```python
from build123d import *

# Parameters (mm, degrees)
BOSS_EXTRUDE1_DEPTH     = 60
CUT_EXTRUDE1_DEPTH      = 144.527000944
CUT_EXTRUDE1_DEPTH_BACK = 3
SKETCH3_R               = 2
CUT_EXTRUDE2_DEPTH      = 4


with BuildPart() as part:
    # Sketch1 → Boss-Extrude1 (new body)
    with BuildSketch(Plane(origin=(0, 0, 0), x_dir=(1, 0, 0), z_dir=(0, 1, 0))):
        Polygon((130, 10), (0, 10), (10, 0), (120, 0), align=None)
    extrude(amount=BOSS_EXTRUDE1_DEPTH)

    # Sketch2 → Cut-Extrude1 (cut, two sides: drawn at the far end of the back side and taken through both)
    with BuildSketch(Plane(origin=(0, 60, 0), x_dir=(1, 0, 0), z_dir=(0, 1, 0)).offset(-CUT_EXTRUDE1_DEPTH_BACK)):
        Polygon((125, 5), (5, 5), (10, 0), (120, 0), align=None)
    extrude(amount=CUT_EXTRUDE1_DEPTH + CUT_EXTRUDE1_DEPTH_BACK, mode=Mode.SUBTRACT)

    # Sketch3 → Cut-Extrude2 (cut)
    with BuildSketch(Plane.XY):
        with Locations((30, 28.5)):
            Circle(SKETCH3_R)
        with Locations((100, 28.5)):
            Circle(SKETCH3_R)
    extrude(amount=-CUT_EXTRUDE2_DEPTH, mode=Mode.SUBTRACT)


solid = part.part
```
Could you check a few things on this model? Use its own coordinates, in mm. A direction names the side the tool comes from. Coordinates: 2 decimals unless noted, no trailing zeros. Write each loop counter-clockwise with the first axis right and the second up, starting at its lowest first coordinate (ties: lowest second). Pieces come first, ordered by that corner, then holes. Notation, with made-up numbers: (81.25, 26) -> (128.25, 26) arc R29 cw to (128.25, 48) -> close; hole circle Ø4 at (60.5, 13.25). An arc over 180 degrees is marked (long way). Return JSON: item names as keys, results as strings.
(1) We'd pull the mould along Y, two halves only. Please class faces 1 (the flat face through (64, 0, -5)), 2 (the flat face through (64, 60, -8)), 3 (the cylindrical face through (30.923, 26.726, -1.972)), 4 (the flat face through (125, 30, -5)): +Y half, -Y half, draft (parallel to the pull), parting line (faces both ways), or undercut.
Numbers:
{"face 1": "-Y half", "face 2": "+Y half", "face 3": "undercut", "face 4": "draft"}
(2) I need wall thicknesses on L1, parallel to Y at x = 30, z = -1.1; L2, parallel to Z at x = 124, y = 8; L3, parallel to Y at x = 32, z = -4.25. Which ranges of each line are inside material? Lowest first, please.
Numbers:
{"L1": "y = 0 to 26.5, 30.5 to 57", "L2": "z = -10 to -4", "L3": "y = 0 to 57"}
(3) Imagine slicing it at C-C, the plane y = 11.5. Please give me the cut outline in (x, z).
Numbers:
{"outline": "(0, -10) -> (130, -10) -> (120, 0) -> (10, 0) -> close"}
(4) I'm going to push flat-ended pins straight in: pin 1 (3.5 mm diameter, centred on x = 46.5, y = 58.5, fed in from +Z); pin 2 (2 mm diameter, centred on x = 30.5, y = 29, fed in from +Z); pin 3 (1.5 mm diameter, centred on x = 91.5, z = -3, fed in from +Y); pin 4 (1 mm diameter, centred on y = 47, z = -5, fed in from +X). Where does each tip first touch, or does it pass through?
Numbers:
{"pin 1": "stops at z = 0", "pin 2": "stops at z = -4", "pin 3": "stops at y = 57", "pin 4": "stops at x = 125.5"}
(5) Imagine slicing it at B-B, the plane z = -1.5. Please give me the cut outline in (x, y), then the cut area to 3 significant figures.
Numbers:
{"outline": "(8.5, 0) -> (121.5, 0) -> (121.5, 57) -> (8.5, 57) -> close; hole circle Ø4 at (30, 28.5); hole circle Ø4 at (100, 28.5)", "area": "6,420 mm2"}
(6) Imagine slicing it at D-D, the plane z = -8.25. Please give me the cut outline in (x, y), then the cut area to 3 significant figures.
Numbers:
{"outline": "(1.75, 0) -> (128.25, 0) -> (128.25, 60) -> (1.75, 60) -> close", "area": "7,590 mm2"}
(7) Which directions (+Z, -Z, +X, -X, +Y, -Y) give clear straight access to the entire face, cutting with the end or side of a thin tool? Please do faces 5 (the flat face through (64, 57, -3)), 6 (the flat face through (66, 30, -10)), 7 (the flat face through (30, 29, -4)).
Numbers:
{"face 5": "+Z, +X, -X, +Y", "face 6": "-Z, +X, -X, +Y, -Y", "face 7": "+Z"}
(8) Imagine slicing it at A-A, the plane x = 100. Please give me the cut outline in (y, z).
Numbers:
{"outline": "(0, -10) -> (60, -10) -> (60, -5) -> (57, -5) -> (57, 0) -> (30.5, 0) -> (30.5, -4) -> (26.5, -4) -> (26.5, 0) -> (0, 0) -> close"}
